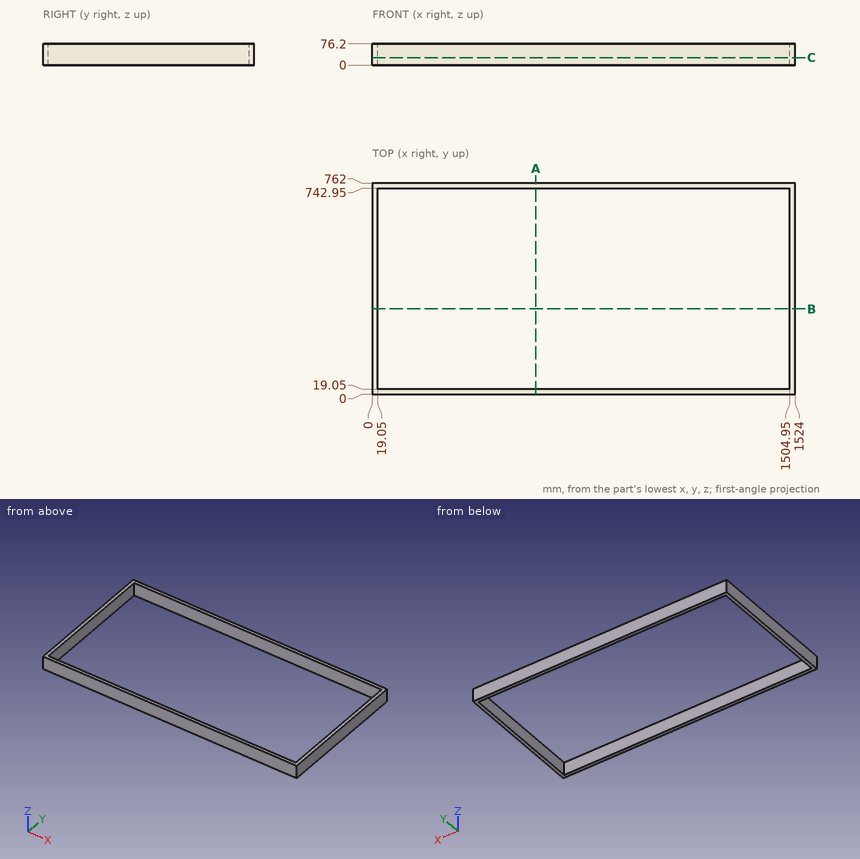
The drawing under review shows one solid part. Ordinate dimensions are in mm from its lowest x, y, z. Give positions to 0.01 mm unless a question says otherwise; leave off trailing zeros. Order: outer loops, then holes, each group sorted by start corner. A loop starts at its lowest first (then second) coordinate and runs counter-clockwise, first axis right, second up. Notation, with made-up numbers: (29.25, 44.25) - (56.25, 44.25) arc R31 ccw to (56.25, 79.25) - close; hole circle Ø6 at (0.25, 58.5). An arc over 180 degrees is marked (long way). Answer as a JSON object with one key per item and string values. Group by question number.
Item 1: Take a section at C-C on z = 27.5. Give the boundary of the cut face in (x, y), and give its area (3 significant figures).
Item 2: Wall thickness on line 1 along X through (y, z) = (477, 17.5); line 2 along Y through (x, z) = (281, 20): over which ranges is each line inside the solid? List them lowest first.
Item 3: Take a section at B-B on y = 308.5. Give the boundary of the cut face in (x, z), and give its area (3 significant figures).
Item 4: Take a section at A-A on x = 589.5. Give the boundary of the cut face in (y, z).
Reported:
{
 "1": {"outline": "(0, 0) - (1524, 0) - (1524, 762) - (0, 762) - close; hole (19.05, 19.05) - (1504.95, 19.05) - (1504.95, 742.95) - (19.05, 742.95) - close", "area": "85,600 mm^2"},
 "2": {"line 1": "0 to 19.05, 1504.95 to 1524", "line 2": "0 to 19.05, 742.95 to 762"},
 "3": {"outline": "(0, 0) - (19.05, 0) - (19.05, 76.2) - (0, 76.2) - close; (1504.95, 0) - (1524, 0) - (1524, 76.2) - (1504.95, 76.2) - close", "area": "2,900 mm^2"},
 "4": {"outline": "(0, 0) - (19.05, 0) - (19.05, 76.2) - (0, 76.2) - close; (742.95, 0) - (762, 0) - (762, 76.2) - (742.95, 76.2) - close"}
}
